Check sheet for the modelled part. Datum: model origin and axes. Units: mm. A direction names the side the tool comes from. Coordinates: 2 decimals unless noted, no trailing zeros. Write each loop counter-clockwise with the first axis right and the second up, starting at its lowest first coordinate (ties: lowest second). Pieces come first, ordered by that corner, then holes. Notation, with made-up numbers: (-20, -28.5) -> (5, -28.5) arc R21 cw to (5, -2.5) -> close; hole circle Ø9 at (-21, -5.75). An arc over 180 degrees is marked (long way). Put each result on its own line as item: value.
```python
from build123d import *

# Parameters (mm, degrees)
SKETCH1_R           = 1.5875
BOSS_EXTRUDE1_DEPTH = 6.35


with BuildPart() as part:
    # Sketch1 → Boss-Extrude1 (new body)
    with BuildSketch(Plane(origin=(0, 0, 0), x_dir=(1, 0, 0), z_dir=(0, 1, 0))):
        with BuildLine():
            Line((-51.235076938, -113.333409223), (246.459341535, -113.333409223))
            Line((246.459341535, -113.333409223), (246.459341535, -37.133409223))
            Line((246.459341535, -37.133409223), (-51.235076938, -37.133409223))
            ThreePointArc((-51.235076938, -37.133409223), (-55.725204999, -38.993281163), (-57.585076938, -43.483409223))
            Line((-57.585076938, -43.483409223), (-57.585076938, -106.983409223))
            ThreePointArc((-57.585076938, -106.983409223), (-55.725204999, -111.473537284), (-51.235076938, -113.333409223))
        make_face()
        with Locations(Location((-51.235076938, -100.633409223, 0), (0, 0, 270))):
            Circle(SKETCH1_R, mode=Mode.SUBTRACT)
        with Locations(Location((-51.235076938, -49.833409223, 0), (0, 0, 270))):
            Circle(SKETCH1_R, mode=Mode.SUBTRACT)
        with Locations(Location((100.787132298, -100.633409223, 0), (0, 0, 270))):
            Circle(SKETCH1_R, mode=Mode.SUBTRACT)
        with Locations(Location((100.787132298, -49.833409223, 0), (0, 0, 270))):
            Circle(SKETCH1_R, mode=Mode.SUBTRACT)
        with Locations(Location((221.059341535, -106.983409223, 0), (0, 0, 270))):
            Circle(SKETCH1_R, mode=Mode.SUBTRACT)
        with Locations(Location((221.059341535, -43.483409223, 0), (0, 0, 270))):
            Circle(SKETCH1_R, mode=Mode.SUBTRACT)
        Polygon((-54.410076938, -75.233409223), (-54.410076938, -62.533409223), (-48.060076938, -62.533409223), (-48.060076938, -87.933409223), (-54.410076938, -87.933409223), align=None, mode=Mode.SUBTRACT)
        Polygon((97.612132298, -75.233409223), (97.612132298, -62.533409223), (103.962132298, -62.533409223), (103.962132298, -87.933409223), (97.612132298, -87.933409223), align=None, mode=Mode.SUBTRACT)
        Polygon((208.359341535, -103.808409223), (202.009341535, -103.808409223), (202.009341535, -110.158409223), (214.709341535, -110.158409223), (214.709341535, -103.808409223), align=None, mode=Mode.SUBTRACT)
        Polygon((208.359341535, -46.658409223), (202.009341535, -46.658409223), (202.009341535, -40.308409223), (214.709341535, -40.308409223), (214.709341535, -46.658409223), align=None, mode=Mode.SUBTRACT)
    extrude(amount=BOSS_EXTRUDE1_DEPTH)


solid = part.part
```
Q1. Cross-section at B-B (y = 1.75). State how many separate pieces and enclosed holes the cut face has, plus the area to 3 significant figures.
Recorded:
separate pieces: 1
enclosed holes: 10
area: 22,600 mm2
Q2. Depth check by flat-ended pin: P1, Ø1.9, axis at x = 100.79, z = 100.63, coming from the -Y side; P2, Ø1.9, axis at x = -52.5, y = 3.5, coming from the +Z side. Enter the tip coordinate at first touch or a pass-through.
Recorded:
P1: passes through
P2: stops at z = 113.33
Q3. Material ranges on line 1 along X through (y, z) = (2.75, 50); line 2 along X through (y, z) = (2.75, 81.5); line 3 along Z through (x, y) = (202.5, 0.5), recorded low to high.
Recorded:
line 1: x = -57.59 to -52.81, -49.66 to 99.21, 102.37 to 246.46
line 2: x = -57.59 to -54.41, -48.06 to 97.61, 103.96 to 246.46
line 3: z = 37.13 to 40.31, 46.66 to 103.81, 110.16 to 113.33
Q4. Mould release check, pull along Z, two halves, no side actions. Record for faces 1 (the flat face through (92, 0, 75)), 2 (the flat face through (214.709, 3, 43)), 3 (the flat face through (96, 3, 113.333)): released by +Z, released by -Z, zero draft, split by the parting line, or undercut.
Recorded:
face 1: zero draft
face 2: undercut
face 3: released by +Z
Q5. Cross-section at A-A (z = 67.5). Record the cut outline in (x, y), plus the area to 3 significant figures.
Recorded:
outline: (-57.59, 0) -> (-54.41, 0) -> (-54.41, 6.35) -> (-57.59, 6.35) -> close; (-48.06, 0) -> (97.61, 0) -> (97.61, 6.35) -> (-48.06, 6.35) -> close; (103.96, 0) -> (246.46, 0) -> (246.46, 6.35) -> (103.96, 6.35) -> close
area: 1,850 mm2
Q6. Tool access check on faces 4 (the flat face through (92, 6.35, 75)), 5 (the flat face through (101, 3, 62.533)). Record the directions out of +Z, -Z, +X, -X, +Y, -Y that give a thin tool (end or side, any length) a straight path to the whole face; none if there is none.
Recorded:
face 4: +Z, -Z, +X, -X, +Y
face 5: +Y, -Y
